```python
from build123d import *

# Parameters (mm, degrees)
SKETCH_1_W          = 138.66
SKETCH_1_H          = 140
EXTRUDE_1_DEPTH     = 140
SKETCH_2_W          = 118.66
SKETCH_2_H          = 100
CUT_EXTRUDE_1_DEPTH = 110
SKETCH_3_W          = 100
SKETCH_3_H          = 13
EXTRUDE_2_DEPTH     = 100
SKETCH_4_R          = 3
CUT_EXTRUDE_3_DEPTH = 220.026594047
SKETCH_5_W          = 12
SKETCH_5_H          = 12
EXTRUDE_3_DEPTH     = 10
SKETCH_6_R          = 14.490887282
SKETCH_6_R_2        = 4.490887282
EXTRUDE_2_2_DEPTH   = 12
SKETCH_7_R          = 4.490887282
CUT_EXTRUDE_4_DEPTH = 269.968786056
EXTRUDE_4_DEPTH     = 10
SKETCH_10_W         = 30
SKETCH_10_H         = 30
CUT_EXTRUDE_6_DEPTH = 40


with BuildPart() as part:
    # 草圖1 → 填料-伸長1 (new body)
    with BuildSketch(Plane(origin=(0, 0, 0), x_dir=(1, 0, 0), z_dir=(0, 1, 0))):
        Rectangle(SKETCH_1_W, SKETCH_1_H)
    extrude(amount=EXTRUDE_1_DEPTH)

    # 草圖2 → 除料-伸長1 (cut)
    with BuildSketch(Plane(origin=(0, 140, 0), x_dir=(1, 0, 0), z_dir=(0, 1, 0))):
        with Locations((-10, 0)):
            Rectangle(SKETCH_2_W, SKETCH_2_H)
    extrude(amount=-CUT_EXTRUDE_1_DEPTH, mode=Mode.SUBTRACT)

    # 草圖3 → Extrude 2 (add)
    with BuildSketch(Plane.ZY.offset(69.33)):
        with Locations((0, 13.5)):
            Rectangle(SKETCH_3_W, SKETCH_3_H)
    extrude(amount=EXTRUDE_2_DEPTH)

    # 草圖4 → 除料-伸長3 (cut, through all)
    with BuildSketch(Plane(origin=(0, 20, 0), x_dir=(1, 0, 0), z_dir=(0, 1, 0))):
        with Locations(Location((-89.33, 0, 0), (0, 0, 270))):
            Circle(SKETCH_4_R)
    extrude(amount=-CUT_EXTRUDE_3_DEPTH, mode=Mode.SUBTRACT)

    # 草圖5 → 填料-伸長3 (add)
    with BuildSketch(Plane(origin=(0, 0, -70), x_dir=(-1, 0, 0), z_dir=(0, 0, -1))):
        with Locations((-28.33, 126)):
            Rectangle(SKETCH_5_W, SKETCH_5_H)
    extrude(amount=EXTRUDE_3_DEPTH)

    # 草圖6 → Extrude 2 2 (add)
    with BuildSketch(Plane(origin=(34.33, 0, 0), x_dir=(0, 0, -1), z_dir=(1, 0, 0))):
        with Locations((82.5, 132)):
            Circle(SKETCH_6_R)
        with Locations((82.5, 132)):
            Circle(SKETCH_6_R_2, mode=Mode.SUBTRACT)
    extrude(amount=-EXTRUDE_2_2_DEPTH)

    # 草圖7 → 除料-伸長4 (cut, through all)
    with BuildSketch(Plane(origin=(34.33, 0, 0), x_dir=(0, 0, -1), z_dir=(1, 0, 0))):
        with Locations((82.5, 132)):
            Circle(SKETCH_7_R)
    extrude(amount=-CUT_EXTRUDE_4_DEPTH, mode=Mode.SUBTRACT)

    # 草圖8 → 填料-伸長4 (add)
    with BuildSketch(Plane.XY.offset(70)):
        with BuildLine():
            Line((69.33, 64.932058031), (69.33, 0))
            Line((69.33, 0), (-69.33, 0))
            Line((-69.33, 0), (-69.33, 59.86))
            add(Edge.make_bspline(
                [(-69.33, 59.86), (-30.324326289, 14.723815627), (-7.370352849, 53.302477249), (5.662490983, 78.887059451), (32.075816325, 96.876157593), (69.33, 64.932058031)],
                knots=[0, 0, 0, 0, 0.759134607, 0.799849306, 1, 1, 1, 1], degree=3))
        make_face()
    extrude(amount=EXTRUDE_4_DEPTH)

    # 草圖10 → 除料-伸長6 (cut)
    with BuildSketch(Plane.ZY.offset(-49.33)):
        with Locations((-11, 110)):
            Rectangle(SKETCH_10_W, SKETCH_10_H)
    extrude(amount=-CUT_EXTRUDE_6_DEPTH, mode=Mode.SUBTRACT)


solid = part.part
```
Design review of the part built by this model. Coordinates are the model's own, in mm. A direction names the side the tool comes from. Give positions to 0.01 mm unless a question says otherwise; leave off trailing zeros. Loops run counter-clockwise (first coordinate to the right, second up) from the corner with the lowest first, then second, coordinate; pieces in that order, holes last. Notation, with made-up numbers: M 52.25,78.25 L 100.25,78.25 A20 ccw 100.25,94.25 Z; hole C -7.5,12 d6. An arc over 180 degrees is marked long. Return JSON: item names as keys, results as strings. Group by question number.
Item 1: We need section A-A (z = -82.5). Give the boundary of the cut face in (x, y), and give its area (3 significant figures).
Item 2: We need section B-B (y = 132). Give the boundary of the cut face in (x, z).
Item 3: Insertion check: pin 1 Ø3 at (y, z) = (74, -30) entering from -X; pin 2 Ø5 at (x, y) = (-11, 37) entering from -Z; pin 3 Ø8 at (y, z) = (126.5, -82.5) entering from +X. Each pin has a flat end and moves straight along its axis. Give the tip position at first contact, or say it passes through.
Item 4: Mouldability with a two-part tool opening along Z and no side actions: class faces 4 (the flat face through (-169.33, 14, -1)), 5 (the cylindrical face through (-92.26, 13.59, -0.65)), 6 (the flat face through (-119, 13, -50)) as released by +Z, released by -Z, zero draft, split by the parting line, or undercut.
Item 5: Tool access review of faces 1 (the flat face through (34.33, 129, -86.3)), 2 (the flat face through (59, 95, -11)), 3 (the flat face through (-11, 30, -1)): name each direction out of +Z, -Z, +X, -X, +Y, -Y from which nothing blocks a thin tool from reaching the whole face with its end or side.
Item 6: For probe 1 along Y at (x, z) = (22.5, -83); probe 2 along Z at (x, y) = (-36.5, 125); probe 3 along Z at (x, y) = (-13.5, 10.5), list the stretches that pass through material, from the lowest coordinate up.
Item 7: We need section C-C (z = 0). Give the boundary of the cut face in (x, y).
Item 8: We need section D-D (z = -46). Give the boundary of the cut face in (x, y).
Output:
{
 "1": {"outline": "M 22.33,117.51 L 34.33,117.51 L 34.33,127.51 L 22.33,127.51 Z; M 22.33,136.49 L 34.33,136.49 L 34.33,146.49 L 22.33,146.49 Z", "area": "240 mm^2"},
 "2": {"outline": "M -69.33,-70 L 22.33,-70 L 22.33,-78.01 L 34.33,-78.01 L 34.33,-70 L 69.33,-70 L 69.33,70 L -69.33,70 L -69.33,50 L 49.33,50 L 49.33,-50 L -69.33,-50 Z; M 22.33,-96.99 L 34.33,-96.99 L 34.33,-86.99 L 22.33,-86.99 Z"},
 "3": {"pin 1": "stops at x = 49.33", "pin 2": "stops at z = -70", "pin 3": "stops at x = 34.33"},
 "4": {"face 4": "zero draft", "face 5": "undercut", "face 6": "released by -Z"},
 "5": {"face 1": "-Z, +X, +Y, -Y", "face 2": "+X, -X", "face 3": "-X, +Y"},
 "6": {"probe 1": "y = 117.52 to 127.54, 136.46 to 146.48", "probe 2": "z = -70 to -50, 50 to 70", "probe 3": "z = -70 to 80"},
 "7": {"outline": "M -169.33,7 L -92.33,7 L -92.33,20 L -169.33,20 Z; M -86.33,7 L -69.33,7 L -69.33,0 L 69.33,0 L 69.33,95 L 49.33,95 L 49.33,30 L -69.33,30 L -69.33,20 L -86.33,20 Z; M 49.33,125 L 69.33,125 L 69.33,140 L 49.33,140 Z"},
 "8": {"outline": "M -169.33,7 L -69.33,7 L -69.33,0 L 69.33,0 L 69.33,140 L 49.33,140 L 49.33,30 L -69.33,30 L -69.33,20 L -169.33,20 Z"}
}
